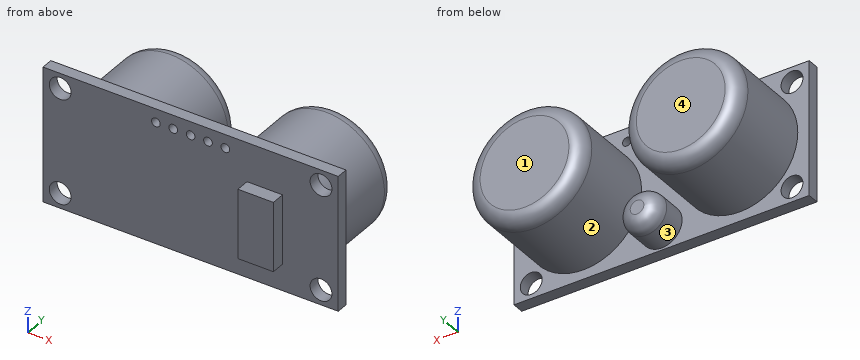
Autodesk Inventor part; units mm, degrees
ref_plane "YZ Plane" through (0, 0, 0) normal (1, 0, 0) x (0, 1, 0)
ref_plane "XZ Plane" through (0, 0, 0) normal (0, 1, 0) x (-1, 0, 0)
ref_plane "XY Plane" through (0, 0, 0) normal (0, 0, 1) x (1, 0, 0)
sketch "Sketch1" plane through (0, 0, 0) normal (0, 1, 0) x (-1, 0, 0)
  line L0 (21.605, -9.85) -> (-21.605, -9.85)
  line L1 (-21.605, -9.85) -> (-21.605, 9.85)
  line L2 (-21.605, 9.85) -> (21.605, 9.85)
  line L3 (21.605, 9.85) -> (21.605, -9.85)
  line L4 (21.605, -9.85) -> (-21.605, 9.85) construction
  line L5 (-21.605, -9.85) -> (21.605, 9.85) construction
  circle A0 centre (-19.084, -7.654) radius 1.6
  circle A1 centre (19.084, 7.654) radius 1.6
  circle A2 centre (-11.43, 0) radius 8.5
  circle A3 centre (11.43, 0) radius 8.5
  circle A4 centre (0, -6.54) radius 3
  circle A5 centre (0, 7.874) radius 0.635
  circle A6 centre (-2.54, 7.874) radius 0.635
  circle A7 centre (-5.08, 7.874) radius 0.635
  circle A8 centre (2.54, 7.874) radius 0.635
  circle A9 centre (5.08, 7.874) radius 0.635
  line L6 (0, -13) -> (0, -21) construction
  line L7 (0, -13) -> (8, -13) construction
  circle A10 centre (-19.084, 7.654) radius 1.6
  circle A11 centre (19.084, -7.654) radius 1.6
  line L8 (-25, 0) -> (-35, 0) construction
  line L9 (-25, 0) -> (-15, 0) construction
  circle A12 centre (0, 6.54) radius 3
  point P0 (0, 0)
  dimension "d0" = 43.21
  dimension "d1" = 19.7
  dimension "d2" = 3.2
  dimension "d5" = 3.2
  dimension "d8" = 17
  dimension "d9" = 17
  dimension "d14" = 6
  dimension "d26" = 1.27
  dimension "d27" = 1.27
  dimension "d28" = 1.27
  dimension "d29" = 1.27
  dimension "d30" = 1.27
  dimension "d31" = 2.54
  dimension "d32" = 2.54
  dimension "d33" = 2.54
  dimension "d34" = 2.54
  dimension "d41" = 22.86
  dimension "d43" = 10.175
  dimension "d44" = 10.175
  dimension "d45" = 6.54
  dimension "d47" = 7.874
  dimension "d48" = 7.654
  dimension "d49" = 7.654
  dimension "d50" = 7.654
  dimension "d51" = 7.654
  dimension "d52" = 90
  dimension "d53" = 180
  dimension "d56" = 2.196
extrude "Extrusion1" add sketch "Sketch1" along normal blind 1.7 contours L0 L1 L2 L3 | A5 | A6 A12 | A6 A12 A8 | A12 A6 | A12 A8 | A8 A12 | A7 | A9 | A10 | A11
extrude "Extrusion2" add sketch "Sketch1" along normal blind 14.6 contours A2 | A3
extrude "Extrusion3" add sketch "Sketch1" along normal blind 7.07 contours A4
sketch "Sketch2" plane through (0, 0, 0) normal (0, -1, 0) x (1, 0, 0)
  line L0 (13.454, 4.1484) -> (8.254, 4.1484)
  line L1 (8.254, 4.1484) -> (8.254, -5.9816)
  line L2 (8.254, -5.9816) -> (13.454, -5.9816)
  line L3 (13.454, -5.9816) -> (13.454, 4.1484)
  line L4 (13.454, 4.1484) -> (8.254, -5.9816) construction
  line L5 (8.254, 4.1484) -> (13.454, -5.9816) construction
  point P0 (0, 0)
  point P1 (10.854, -0.9166)
  dimension "d22" = 5.2
  dimension "d23" = 10.13
extrude "Extrusion4" add sketch "Sketch2" along normal blind 2
extrude "Extrusion5" cut sketch "Sketch1" along normal through all contours A5 | A6 A12 | A12 A6 | A12 A8 | A8 A12 | A7 | A9
fillet "Fillet1" radius 2 2 edges at (19.93, 14.6, 0) (-2.93, 14.6, 0)
fillet "Fillet2" radius 2 1 edges at (3, 7.07, -6.54)
extrude "Extrusion6" cut sketch "Sketch1" along normal through all contours A10 | A11
sketch "Sketch3" plane through (0, 0, 0) normal (0, -1, 0) x (1, 0, 0)
  circle A0 centre (0, 6.54) radius 3
  point P0 (0, 0)
properties part number "srf08"
Work out the finished part from the listing and answer in its coordinate system (mm). Face numbers are marked on the shaded views. A direction names the side the tool comes from. Give positions to 0.01 mm unless a question says otherwise; leave off trailing zeros. Loops run counter-clockwise (first coordinate to the right, second up) from the corner with the lowest first, then second, coordinate; pieces in that order, holes last. Notation, with made-up numbers: (41, -31) - (81, -31) arc R12 ccw to (81, -25) - close; hole circle Ø3 at (70, 7). An arc over 180 degrees is marked (long way). Answer in a Markdown table with one row per item. Add a question column.
Q1. Each of these flat-tipped pins is pushed along its axis until it touches: P1, Ø5, axis at x = -16, y = 9, coming from the +Z side; P2, Ø5, axis at x = 8, y = 8, coming from the -Z side; P3, Ø1.1, axis at x = 2.54, z = 7.874, coming from the +Y side; P4, Ø8, axis at y = 8, z = 1, coming from the -X side. Where does it stop, or does it pass through?
Q2. The part is cut by section D-D (y = 13.25). Determine the outline of the cut face in (x, z).
Q3. The part is cut by section A-A (x = 11.43). Determine the outline of the cut face in (y, z).
Q4. The part is cut by section B-B (y = 9). Determine the outline of the cut face in (x, z), and give its area (3 significant figures).
Q5. The part is cut by section C-C (x = -11.43). Determine the outline of the cut face in (y, z), and give its area (3 significant figures).
Q6. Consider line 1 along Y through (x, z) = (-4, 8.75); line 2 along Z through (x, y) = (0, 1.1); line 3 along X through (y, z) = (7.75, 4.5). Determine where each line is inside the solid, lowest interval first.
Q7. Determine the mould class of the marked faces 1 and 2 for opening direction X: released by +X, released by -X, zero draft, split by the parting line, or undercut.
Q8. A tool of negligible diameter and unlimited length cuts with its end or side. For the marked faces 3 and 4, from which of +Z, -Z, +X, -X, +Y, -Y can it reach the whole face along a straight path? Write none if from no direction.
Solution:
| question | item | result |
|---|---|---|
| 1 | P1 | stops at z = 8.24 |
| 1 | P2 | stops at z = -8.45 |
| 1 | P3 | passes through |
| 1 | P4 | stops at x = -19.93 |
| 2 | outline | circle Ø16.78 at (-11.43, 0); circle Ø16.78 at (11.43, 0) |
| 3 | outline | (-2, -5.98) - (0, -5.98) - (0, -9.85) - (1.7, -9.85) - (1.7, -8.5) - (12.6, -8.5) arc R2 ccw to (14.6, -6.5) - (14.6, 6.5) arc R2 ccw to (12.6, 8.5) - (1.7, 8.5) - (1.7, 9.85) - (0, 9.85) - (0, 4.15) - (-2, 4.15) - close |
| 4 | outline | circle Ø17 at (-11.43, 0); circle Ø17 at (11.43, 0) |
| 4 | area | 454 mm² |
| 5 | outline | (0, -9.85) - (1.7, -9.85) - (1.7, -8.5) - (12.6, -8.5) arc R2 ccw to (14.6, -6.5) - (14.6, 6.5) arc R2 ccw to (12.6, 8.5) - (1.7, 8.5) - (1.7, 9.85) - (0, 9.85) - close |
| 5 | area | 251 mm² |
| 6 | line 1 | y = 0 to 1.7 |
| 6 | line 2 | z = -9.85 to 7.24, 8.51 to 9.85 |
| 6 | line 3 | x = -18.64 to -4.22, 4.22 to 18.64 |
| 7 | face 1 | zero draft |
| 7 | face 2 | undercut |
| 8 | face 3 | +Y |
| 8 | face 4 | +Z, -Z, +X, -X, +Y |
